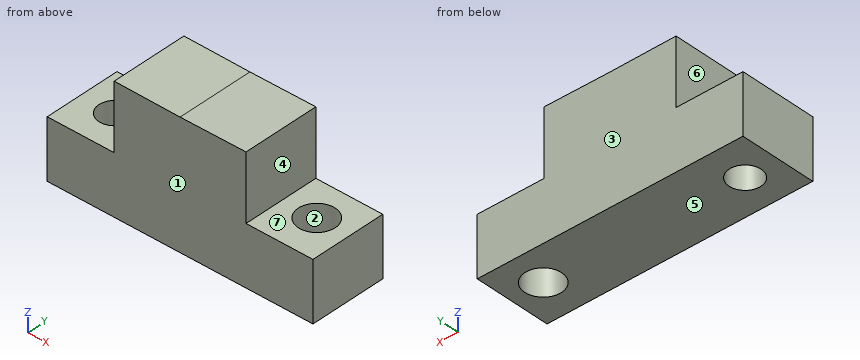
from build123d import *

# Parameters (mm, degrees)
F1_DEPTH = 25.4
F3_DEPTH = 25.4
F4_R     = 6.100082
F6_DEPTH = 50.8
F2_R     = 5.287895
F8_DEPTH = 25.4


with BuildPart() as f1:
    # F0 (on Front) → F1 (new body)
    with BuildSketch(Plane.XZ):
        Polygon((0, 21.703117), (0, 0), (-22.189008, 0), (-22.189008, -19.597592), (10.689595, -19.597592), (21.865079, -19.597592), (21.865079, 21.541156), align=None)
    extrude(amount=F1_DEPTH)

    # F0 (on Front) → F3 (join)
    with BuildSketch(Plane.XZ):
        Polygon((0, 21.703117), (0, 0), (-22.189008, 0), (-22.189008, -19.597592), (10.689595, -19.597592), (21.865079, -19.597592), (21.865079, 21.541156), align=None)
        Polygon((43.730158, 21.703117), (21.865079, 21.541156), (21.865079, -19.597592), (33.040564, -19.597592), (65.919166, -19.597592), (65.919166, 0), (43.730158, 0), align=None)
    extrude(amount=F3_DEPTH)

    # F4 (on Top) → F6 (cut)
    with BuildSketch(Plane.XY):
        with Locations((54.988019, -12.019237)):
            Circle(F4_R)
    extrude(amount=-F6_DEPTH, mode=Mode.SUBTRACT)

    # F2 (on Top) → F8 (cut)
    with BuildSketch(Plane.XY):
        with Locations((-10.94509, -13.110346)):
            Circle(F2_R)
    extrude(amount=-F8_DEPTH, mode=Mode.SUBTRACT)


solid = f1.part
Geometry check sheet. Reference: the model listing, model coordinates, mm. Face numbers are marked on the shaded views. A direction names the side the tool comes from. Round coordinates to 2 decimals unless told otherwise and drop trailing zeros. Order: outer loops, then holes, each group sorted by start corner. A loop starts at its lowest first (then second) coordinate and runs counter-clockwise, first axis right, second up. Notation, with made-up numbers: M 48,-28 L 81,-28 A23 cw 81,8 Z; hole C 36.5,-24 d1. An arc over 180 degrees is marked long. Write each question's results on one line, items separated by ' | '. Start each with the question number.
1. Set-up check for the marked faces 5, 6 and 7: record each of +Z, -Z, +X, -X, +Y, -Y from which the full face is reachable in a straight line by a thin tool's end or side.
2. Material ranges on L1, parallel to X at y = -14.75, z = -16; L2, parallel to X at y = -19.5, z = 1; L3, parallel to Z at x = 2, y = -9.5, recorded low to high. Write a range as from..to.
3. Go/stop test with flat-tipped pins: P1, Ø6.5, axis at y = -12.5, z = 12.5, coming from the +X side; P2, Ø8.5, axis at x = -10.95, y = -13.11, coming from the +Z side; P3, Ø4, axis at x = 26.5, z = -12, coming from the +Y side; P4, Ø12, axis at y = -21, z = 9.5, coming from the -X side. Record where each tip stops, or that it passes through.
4. Cross-section at A-A on y = -16.5. Record the boundary of the cut face in (x, z).
5. Cross-section at B-B on y = -21.25. Record the boundary of the cut face in (x, z).
6. Cross-section at D-D on z = -16.5. Record the boundary of the cut face in (x, y), plus the area to 3 significant figures.
7. Cross-section at C-C on x = -8.5. Record the boundary of the cut face in (y, z).
8. Draft check along Y on the marked faces 1, 2, 3 and 4. Enter one of: pulls with the +Y half, pulls with the -Y half, needs draft (parallel to the pull), parting line crosses it, or undercut.
Resolved:
1) face 5: -Z, +X, -X, +Y, -Y | face 6: +Z, -X, +Y, -Y | face 7: +Z, +X, +Y, -Y
2) L1: -22.19..-15.97, -5.92..49.53, 60.44..65.92 | L2: 0..43.73 | L3: -19.6..21.69
3) P1: x = 43.73 | P2: through | P3: y = 0 | P4: x = 0
4) outline: M -22.19,-19.6 L -15,-19.6 L -15,0 L -22.19,0 Z; M -6.89,-19.6 L 50.85,-19.6 L 50.85,0 L 43.73,0 L 43.73,21.7 L 21.87,21.54 L 0,21.7 L 0,0 L -6.89,0 Z; M 59.13,-19.6 L 65.92,-19.6 L 65.92,0 L 59.13,0 Z
5) outline: M -22.19,-19.6 L 65.92,-19.6 L 65.92,0 L 43.73,0 L 43.73,21.7 L 21.87,21.54 L 0,21.7 L 0,0 L -22.19,0 Z
6) outline: M -22.19,-25.4 L 65.92,-25.4 L 65.92,0 L -22.19,0 Z; hole C -10.95,-13.11 d10.58; hole C 54.99,-12.02 d12.2 | area: 2,030 mm2
7) outline: M -25.4,-19.6 L -17.8,-19.6 L -17.8,0 L -25.4,0 Z; M -8.42,-19.6 L 0,-19.6 L 0,0 L -8.42,0 Z
8) face 1: pulls with the -Y half | face 2: undercut | face 3: pulls with the +Y half | face 4: needs draft
